Design review of the part shown in the three views and the two pictorial views. Dimensions are in mm from the part's minimum x, y and z. Round coordinates to 2 decimals unless told otherwise and drop trailing zeros. Loops run counter-clockwise (first coordinate to the right, second up) from the corner with the lowest first, then second, coordinate; pieces in that order, holes last. Notation, with made-up numbers: (35.5, 84.25) -> (58.5, 84.25) arc R31 cw to (58.5, 114.25) -> close; hole circle Ø6 at (82, -1.5). An arc over 180 degrees is marked (long way). Return JSON: item names as keys, results as strings. Group by question number.
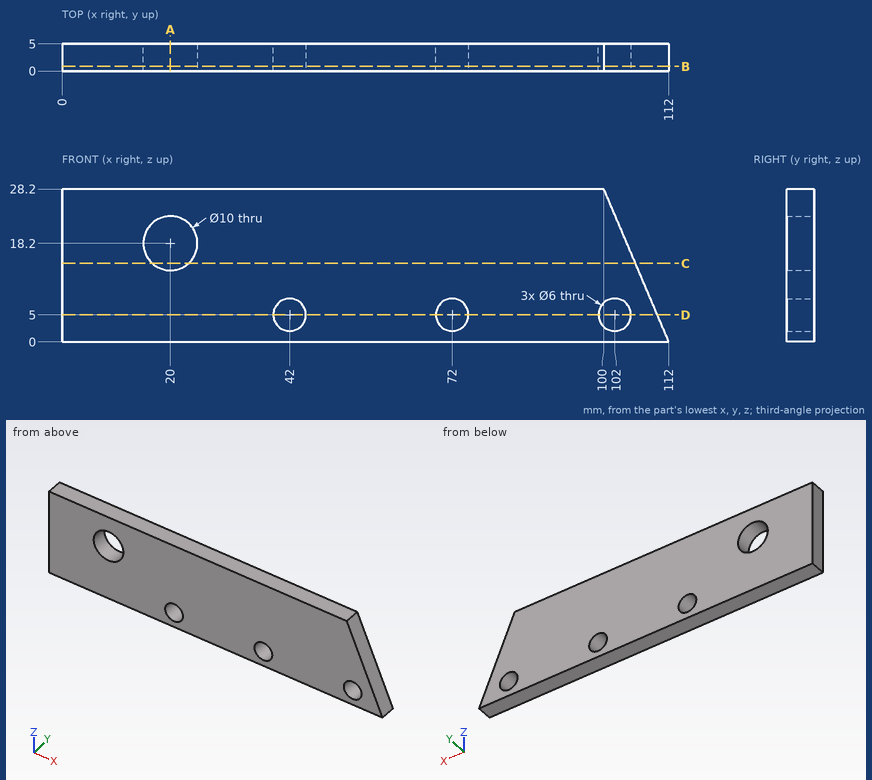
1. Wall thickness on line 1 (Z direction, x = 20, y = 2.65); line 2 (Z direction, x = 72, y = 0.95); line 3 (X direction, y = 4.55, z = 20.5): over which ranges is each line inside the solid? List them lowest first.
2. We need section C-C, the plane z = 14.5. Write out the cut boundary in (x, y), then the cut area to 3 significant figures.
3. We need section B-B, the plane y = 0.85. Write out the cut boundary in (x, z), then the cut area to 3 significant figures.
4. We need section D-D, the plane z = 5. Write out the cut boundary in (x, y), then the cut area to 3 significant figures.
5. We need section A-A, the plane x = 20. Write out the cut boundary in (y, z).
Check sheet entries:
{
 "1": {"line 1": "z = 0 to 13.2, 23.2 to 28.2", "line 2": "z = 0 to 2, 8 to 28.2", "line 3": "x = 0 to 15.56, 24.44 to 103.28"},
 "2": {"outline": "(0, 0) -> (16.64, 0) -> (16.64, 5) -> (0, 5) -> close; (23.36, 0) -> (105.83, 0) -> (105.83, 5) -> (23.36, 5) -> close", "area": "496 mm²"},
 "3": {"outline": "(0, 0) -> (112, 0) -> (100, 28.2) -> (0, 28.2) -> close; hole circle Ø10 at (20, 18.2); hole circle Ø6 at (42, 5); hole circle Ø6 at (72, 5); hole circle Ø6 at (102, 5)", "area": "2,830 mm²"},
 "4": {"outline": "(0, 0) -> (39, 0) -> (39, 5) -> (0, 5) -> close; (45, 0) -> (69, 0) -> (69, 5) -> (45, 5) -> close; (75, 0) -> (99, 0) -> (99, 5) -> (75, 5) -> close; (105, 0) -> (109.87, 0) -> (109.87, 5) -> (105, 5) -> close", "area": "459 mm²"},
 "5": {"outline": "(0, 0) -> (5, 0) -> (5, 13.2) -> (0, 13.2) -> close; (0, 23.2) -> (5, 23.2) -> (5, 28.2) -> (0, 28.2) -> close"}
}
